Source: CAD feature listing. Evaluate the final solid. Frame: model axes, mm. Face numbers are marked on the shaded views. A direction names the side the tool comes from. Round coordinates to 2 decimals unless told otherwise and drop trailing zeros. Loops run counter-clockwise (first coordinate to the right, second up) from the corner with the lowest first, then second, coordinate; pieces in that order, holes last. Notation, with made-up numbers: M 74.25,66.5 L 129.25,66.5 A12 ccw 129.25,82.5 Z; hole C 83.25,7.5 d3. An arc over 180 degrees is marked long. Answer as a JSON object with one key per item and string values.
Autodesk Fusion 360 part; units mm, degrees
sketch "Sketch1" plane through (0, 0, 0) normal (0, 0, 1) x (1, 0, 0)
  line L0 (18.5, -17.5) -> (-18.5, -17.5)
  line L1 (-18.5, -17.5) -> (-18.5, 17.5)
  line L2 (-18.5, 17.5) -> (18.5, 17.5)
  line L3 (18.5, 17.5) -> (18.5, -17.5)
  line L4 (18.5, -17.5) -> (-18.5, 17.5) construction
  line L5 (-18.5, -17.5) -> (18.5, 17.5) construction
  dimension "d1" = 35
  dimension "d2" = 37
extrude "Extrude1" add sketch "Sketch1" along normal blind 20
sketch "Sketch4" plane through (18.5, 0, 0) normal (1, 0, 0) x (0, 1, 0)
  line L0 (-17.5, 0) -> (17.5, 0)
  line L1 (17.5, 0) -> (17.5, 20)
  line L2 (17.5, 20) -> (-17.5, 20)
  line L3 (-17.5, 20) -> (-17.5, 0)
  line L4 (12.5, 3) -> (-12.5, 3)
  line L5 (-12.5, 3) -> (-12.5, 17)
  line L6 (-12.5, 17) -> (12.5, 17)
  line L7 (12.5, 17) -> (12.5, 3)
  line L8 (12.5, 3) -> (-12.5, 17) construction
  line L9 (-12.5, 3) -> (12.5, 17) construction
  point P0 (0, 10)
  dimension "d39" = 25
  dimension "d40" = 14
  dimension "d41" = 10
extrude "Extrude3" cut sketch "Sketch4" against normal blind 17 contours L4 L5 L6 L7
sketch "Sketch5" plane through (18.5, 0, 0) normal (1, 0, 0) x (0, 1, 0)
  line L0 (-12.5, 3) -> (-12.5, 17)
  line L1 (-12.5, 17) -> (12.5, 17)
  line L2 (12.5, 17) -> (12.5, 3)
  line L3 (12.5, 3) -> (-12.5, 3)
  line L4 (-17.5, 0) -> (17.5, 0)
  line L5 (17.5, 0) -> (17.5, 20)
  line L6 (17.5, 20) -> (-17.5, 20)
  line L7 (-17.5, 20) -> (-17.5, 0)
  point P0 (-14, 10)
  point P1 (14, 10)
  dimension "d44" = 1.5
  dimension "d45" = 1.5
  dimension "d46" = 10
  dimension "d47" = 10
hole "Hole3" at (18.5, -14, 10) at (18.5, 14, 10) direction (-1, 0, 0) diameter 1.623 depth 6 tip angle 118
hole "Hole4" at (8.5, 17.5, 10) direction (0, -1, 0) diameter 12 depth 5 tip angle 180
sketch "Sketch6" plane through (0, 0, 20) normal (0, 0, 1) x (-1, 0, 0)
  line L0 (-18.5, -17.5) -> (18.5, -17.5)
  line L1 (18.5, -17.5) -> (18.5, 17.5)
  line L2 (18.5, 17.5) -> (-18.5, 17.5)
  line L3 (-18.5, 17.5) -> (-18.5, -17.5)
  line L4 (15.5, -12.5) -> (1.5, -12.5)
  line L5 (1.5, -12.5) -> (1.5, 12.5)
  line L6 (1.5, 12.5) -> (15.5, 12.5)
  line L7 (15.5, 12.5) -> (15.5, -12.5)
  point P0 (15.5, 0)
  dimension "d58" = 14
  dimension "d59" = 25
  dimension "d60" = 20
  dimension "d61" = 17.5
extrude "Extrude4" cut sketch "Sketch6" against normal blind 17 contours L4 L5 L6 L7
sketch "Sketch7" plane through (0, 0, 20) normal (0, 0, 1) x (-1, 0, 0)
  line L0 (1.5, -12.5) -> (1.5, 12.5)
  line L1 (1.5, 12.5) -> (15.5, 12.5)
  line L2 (15.5, 12.5) -> (15.5, -12.5)
  line L3 (15.5, -12.5) -> (1.5, -12.5)
  line L4 (-18.5, -17.5) -> (18.5, -17.5)
  line L5 (18.5, -17.5) -> (18.5, 17.5)
  line L6 (18.5, 17.5) -> (-18.5, 17.5)
  line L7 (-18.5, 17.5) -> (-18.5, -17.5)
  point P0 (8.5, 14)
  point P1 (8.5, -14)
  dimension "d64" = 1.5
  dimension "d65" = 1.5
  dimension "d66" = 7
  dimension "d67" = 7
hole "Hole5" at (-8.5, -14, 20) at (-8.5, 14, 20) direction (0, 0, -1) diameter 1.623 depth 6 tip angle 118
hole "Hole6" at (-8.5, 17.5, 10) direction (0, -1, 0) diameter 12 depth 5 tip angle 180
fillet "Fillet3" radius 0.5 10 edges at (18.5, -12.5, 10) (18.5, 0, 17) (18.5, 12.5, 10) (18.5, 0, 3) (10.6697, 17.5, 4.406) (-6.3303, 17.5, 4.406) (-1.5, 0, 20) (-8.5, 12.5, 20) (-15.5, 0, 20) (-8.5, -12.5, 20)
fillet "Fillet4" radius 1 12 edges at (-18.5, 0, 20) (0, -17.5, 20) (-18.5, -17.5, 10) (18.5, 0, 20) (0, 17.5, 20) (18.5, -17.5, 10) (0, -17.5, 0) (-18.5, 0, 0) (-18.5, 17.5, 10) (0, 17.5, 0) (18.5, 17.5, 10) (18.5, 0, 0)
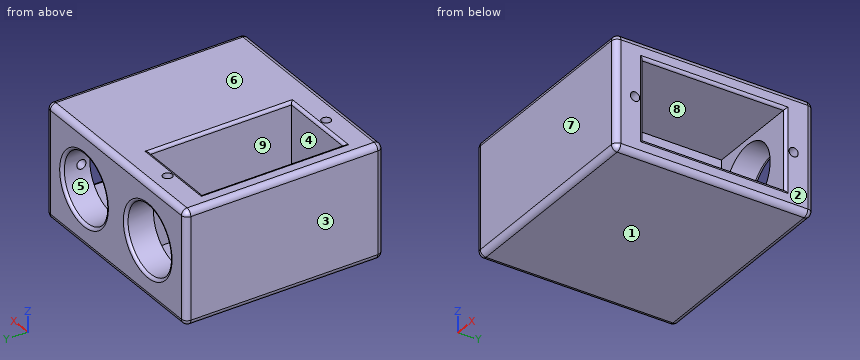
Item 1: Pull-direction query (X, two-part tool) for the marked faces 1, 2, 3 and 4; classes: pulls with the +X half, pulls with the -X half, needs draft (parallel to the pull), parting line crosses it, or undercut.
Answer sheet:
{"face 1": "needs draft", "face 2": "pulls with the +X half", "face 3": "pulls with the -X half", "face 4": "undercut"}
Item 2: Access query for the marked faces 5, 6, 7, 8 and 9. Directions: +Z, -Z, +X, -X, +Y, -Y. A direction counts if a zero-diameter tool reaches every point of the face in a straight line with its end or side. Return the directions, or none.
Answer sheet:
{"face 5": "+Y", "face 6": "+Z, +X, -X, +Y, -Y", "face 7": "+Z, -Z, +X, -X, -Y", "face 8": "+X", "face 9": "+Z"}
Item 3: Line query: probe 1 along Y at (x, z) = (15.95, 10); probe 2 along X at (y, z) = (15.7, 10); probe 3 along Y at (x, z) = (15.5, 7.5). Output: solid intervals per line, ascending. Write a range as from..to.
Answer sheet:
{"probe 1": "y = -17.5..-14.81, -13.19..-12.5, 12.5..13.19, 14.81..17.5", "probe 2": "x = -18.5..-14.5, -2.5..2.5, 14.5..18.5", "probe 3": "y = -17.5..-12.5, 12.5..17.5"}
Item 4: Contact query for flat-ended pins moving along their axis: pin 1 Ø7 at (x, y) = (-10, -3.5) entering from +Z; pin 2 Ø4 at (y, z) = (-2, 9) entering from +X; pin 3 Ø1.3 at (y, z) = (-14, 10) entering from +X. Output: stop coordinate, or through.
Answer sheet:
{"pin 1": "stops at z = 3", "pin 2": "stops at x = 1.5", "pin 3": "stops at x = 12.4"}
Item 5: Section A-A on y = -3.5. Return the cut outline in (x, z), then the cut area to 3 significant figures.
Answer sheet:
{"outline": "M -18.5,1 A1 ccw -17.5,0 L 17.5,0 A1 ccw 18.5,1 L 18.5,2.5 A0.5 ccw 18,3 L 1.5,3 L 1.5,17 L 18,17 A0.5 ccw 18.5,17.5 L 18.5,19 A1 ccw 17.5,20 L -1,20 A0.5 ccw -1.5,19.5 L -1.5,3 L -15.5,3 L -15.5,19.5 A0.5 ccw -16,20 L -17.5,20 A1 ccw -18.5,19 Z", "area": "263 mm²"}
Item 6: Section B-B on x = 8.5. Return the cut outline in (y, z).
Answer sheet:
{"outline": "M -17.5,1 A1 ccw -16.5,0 L 16.5,0 A1 ccw 17.5,1 L 17.5,3.5 A0.5 ccw 17,4 L 12.5,4 L 12.5,3 L -12.5,3 L -12.5,17 L 12.5,17 L 12.5,16 L 17,16 A0.5 ccw 17.5,16.5 L 17.5,19 A1 ccw 16.5,20 L -16.5,20 A1 ccw -17.5,19 Z"}
Item 7: Section C-C on z = 15.5. Give the number of separate pieces and of enclosed holes in the cut face, then the cut area to 3 significant figures.
Answer sheet:
{"separate pieces": "2", "enclosed holes": "1", "area": "469 mm²"}
